Part model, mm, in its own coordinate system. A direction names the side the tool comes from. Coordinates: 2 decimals unless noted, no trailing zeros. Use a Markdown table: item, result. Add a question column.
Q1. Tool access for faces 5 (the flat face through (108, 177.843, 0)), 6 (the flat face through (82, 206.827, 0)), 7 (the cylindrical face through (93.662, 192.694, 25.287)): list every direction of +Z, -Z, +X, -X, +Y, -Y with a clear straight run to the whole face (end or side of a thin tool).
Q2. Mould opens along Z. For faces 1 (the flat face through (94, 165.143, -5)), 2 (the cylindrical face through (80.775, 213.266, -0.344)), 3 (the cylindrical face through (96.384, 192.694, -24.484)), 4 (the flat face through (82, 177.843, 0)) say: released by +Z, released by -Z, zero draft, split by the parting line, or undercut.
Q3. Pin check, flat tips, straight feed: pin 1 Ø1 at (x, z) = (108, 0.5) entering from +Y; pin 2 Ø1.5 at (x, z) = (150, 18.5) entering from +Y; pin 3 Ø6 at (x, y) = (130.5, 207) entering from +Z; pin 4 Ø8 at (x, y) = (143.5, 186) entering from -Z. Stop position of each tip, or through.
Q4. Wall check: L1, parallel to X at y = 174, z = 0; L2, parallel to X at y = 178, z = 0; L3, parallel to X at y = 195.5, z = 9. Give the ranges that are in metal, low to high. Write a range as from..to.
from build123d import *

# Parameters (mm, degrees)
BOSS_EXTRUDE1_DEPTH      = 28.575
BOSS_EXTRUDE1_DEPTH_BACK = 28.575
SKETCH1_W                = 190.049903163
SKETCH1_H                = 54.384002277
SKETCH2_W                = 210.421602417
SKETCH2_H                = 85.92215432
CUT_EXTRUDE1_DEPTH       = 200.732611311
SKETCH3_R                = 3.175
CUT_EXTRUDE2_DEPTH       = 200.28936731
FILLET1_R                = 2.54
FILLET2_R                = 1.5875
SKETCH4_R                = 1.5875
CUT_EXTRUDE3_DEPTH       = 12.7
CUT_EXTRUDE4_START       = -12.7
SKETCH5_R                = 1.5875
CUT_EXTRUDE4_DEPTH       = 12.7


with BuildPart() as part:
    # Sketch1 → Boss-Extrude1 (new, two sides: drawn at the far end of the back side and taken through both)
    with BuildSketch(Plane.XY.offset(-BOSS_EXTRUDE1_DEPTH_BACK)):
        with Locations((95.024951582, 192.335070701)):
            Rectangle(SKETCH1_W, SKETCH1_H)
    extrude(amount=BOSS_EXTRUDE1_DEPTH + BOSS_EXTRUDE1_DEPTH_BACK)

    # Sketch2 → Cut-Extrude1 (cut, through all)
    with BuildSketch(Plane(origin=(0, 219.527071839, 0), x_dir=(1, 0, 0), z_dir=(0, 1, 0))):
        with Locations((94.245612314, -0.876756677)):
            Rectangle(SKETCH2_W, SKETCH2_H)
        with BuildLine():
            Line((0, 1.5875), (0, -1.5875))
            ThreePointArc((0, -1.5875), (95.024951582, -25.291629574), (190.049903163, -1.5875))
            Line((190.049903163, -1.5875), (190.049903163, 1.5875))
            ThreePointArc((190.049903163, 1.5875), (95.024951582, 24.488158935), (0, 1.5875))
        make_face(mode=Mode.SUBTRACT)
    extrude(amount=-CUT_EXTRUDE1_DEPTH, mode=Mode.SUBTRACT)

    # Sketch3 → Cut-Extrude2 (cut, through all)
    with BuildSketch(Plane(origin=(0, 219.527071839, 0), x_dir=(1, 0, 0), z_dir=(0, 1, 0))):
        with Locations(Location((95.024951582, 0, 0), (0, 0, 270))):
            Circle(SKETCH3_R)
    extrude(amount=-CUT_EXTRUDE2_DEPTH, mode=Mode.SUBTRACT)

    # Fillet1
    fillet1_edges = [part.edges().sort_by_distance(p)[0] for p in [
        (190.049903163, 192.3350707, -1.5875),
        (190.049903163, 192.3350707, 1.5875),
        (0, 192.3350707, 1.5875),
        (0, 192.3350707, -1.5875),
    ]]
    fillet(fillet1_edges, radius=FILLET1_R)

    # Fillet2
    fillet2_edges = [part.edges().sort_by_distance(p)[0] for p in [
        (190.049903163, 165.143069562, 0.013840704),
        (190.049903163, 219.527071839, 0.013840704),
        (95.024951582, 219.527071839, -24.488158935),
        (0, 219.527071839, 0.013840704),
        (95.024951582, 219.527071839, 25.291629574),
        (0.367643144, 219.527071839, 1.371374897),
        (0.378145075, 219.527071839, -1.36087226),
        (189.68226002, 219.527071839, 1.371374897),
        (189.671758089, 219.527071839, -1.36087226),
        (95.024951582, 165.143069562, -24.488158935),
        (0, 165.143069562, 0.013840704),
        (95.024951582, 165.143069562, 25.291629574),
        (0.367643144, 165.143069562, 1.371374897),
        (0.378145075, 165.143069562, -1.36087226),
        (189.68226002, 165.143069562, 1.371374897),
        (189.671758089, 165.143069562, -1.36087226),
    ]]
    fillet(fillet2_edges, radius=FILLET2_R)

    # Sketch4 → Cut-Extrude3 (cut)
    with BuildSketch(Plane(origin=(0, 219.527071839, 0), x_dir=(1, 0, 0), z_dir=(0, 1, 0))):
        with Locations(Location((107.724951582, 0, 0), (0, 0, 270))):
            Circle(SKETCH4_R)
        with Locations(Location((82.324951582, 0, 0), (0, 0, 270))):
            Circle(SKETCH4_R)
    extrude(amount=-CUT_EXTRUDE3_DEPTH, mode=Mode.SUBTRACT)

    # Sketch5 → Cut-Extrude4 (cut)
    with BuildSketch(Plane.XZ.offset(-165.143069562).offset(CUT_EXTRUDE4_START)):
        with Locations(Location((82.324951582, 0, 0), (0, 0, 90))):
            Circle(SKETCH5_R)
        with Locations(Location((107.724951582, 0, 0), (0, 0, 90))):
            Circle(SKETCH5_R)
    extrude(amount=CUT_EXTRUDE4_DEPTH, mode=Mode.SUBTRACT)


solid = part.part
Recorded:
| question | item | result |
|---|---|---|
| 1 | face 5 | -Y |
| 1 | face 6 | +Y |
| 1 | face 7 | +Z, +Y, -Y |
| 2 | face 1 | zero draft |
| 2 | face 2 | undercut |
| 2 | face 3 | released by -Z |
| 2 | face 4 | undercut |
| 3 | pin 1 | y = 206.83 |
| 3 | pin 2 | through |
| 3 | pin 3 | z = 22.67 |
| 3 | pin 4 | z = -19.69 |
| 4 | L1 | 0..80.74, 83.91..91.85, 98.2..106.14, 109.31..190.05 |
| 4 | L2 | 0..91.85, 98.2..190.05 |
| 4 | L3 | 15.48..174.57 |
